Design review of the part built by this model. Coordinates are the model's own, in mm. A direction names the side the tool comes from. Round coordinates to 2 decimals unless told otherwise and drop trailing zeros. Write each loop counter-clockwise with the first axis right and the second up, starting at its lowest first coordinate (ties: lowest second). Pieces come first, ordered by that corner, then holes. Notation, with made-up numbers: (6, -32) -> (21, -32) arc R17 ccw to (21, -18) -> close; hole circle Ø9 at (46.5, 22). An arc over 180 degrees is marked (long way). Write item = value, one per line. Start each with the question number.
Item 1: For pin 1 Ø1.5 at (x, z) = (23, 2) entering from +Y; pin 2 Ø1.9 at (x, z) = (122, 4.5) entering from +Y; pin 3 Ø5.5 at (x, y) = (147.955, 6.35) entering from -Z, all flat-tipped, find the tip position at first contact; note any pin that passes through.
Item 2: Add section C-C, the plane z = 4.5. State the section outline as (x, y) points (3 decimals).
Item 3: To check wall thickness, follow L1, parallel to Y at x = 139.7, z = 4.5; L2, parallel to Y at x = -20, z = 1.5; L3, parallel to X at y = 12, z = 1.5. State the ranges of each line that lie inside material, in increasing order.
Item 4: Machinability: for faces 1 (the flat face through (152.4, -44, 3)), 2 (the flat face through (110, 12.7, 3)), 3 (the flat face through (-111, 12.7, 3)), which of the approach directions +Z, -Z, +X, -X, +Y, -Y give a long, thin tool a straight path to every point of the face, cutting with its end or side? Answer none if there is none.
Item 5: Mouldability with a two-part tool opening along Y and no side actions: class faces 4 (the flat face through (-152.4, -45, 3)), 5 (the cylindrical face through (21.199, 6.676, 3.131)), 6 (the cylindrical face through (41.16, 16.5, 3.13)) as released by +Y, released by -Y, zero draft, split by the parting line, or undercut.
Item 6: Add section A-A, the plane x = 0. State the section outline as (y, z) points (3 decimals).
Item 7: Add section D-D, the plane x = -118. State the section outline as (y, z) points.
Item 8: Add section B-B, the plane y = 0. State the section outline as (x, z) points (3 decimals).
from build123d import *

# Parameters (mm, degrees)
SKETCH1_R           = 22.225
BOSS_EXTRUDE1_DEPTH = 6.35
SKETCH2_R           = 2.159
CUT_EXTRUDE1_DEPTH  = 7.35


with BuildPart() as part:
    # Sketch1 → Boss-Extrude1 (new body)
    with BuildSketch(Plane.XY):
        with BuildLine():
            Line((-152.4, 12.7), (-68.685751798, 12.7))
            ThreePointArc((-68.685751798, 12.7), (-41.532009619, 16.395790255), (-16.353750428, 27.214285714))
            ThreePointArc((-16.353750428, 27.214285714), (0, 31.75), (16.353750428, 27.214285714))
            ThreePointArc((16.353750428, 27.214285714), (41.532009619, 16.395790255), (68.685751798, 12.7))
            Line((68.685751798, 12.7), (152.4, 12.7))
            Line((152.4, 12.7), (152.4, -101.6))
            Line((152.4, -101.6), (-152.4, -101.6))
            Line((-152.4, -101.6), (-152.4, 12.7))
        make_face()
        Circle(SKETCH1_R, mode=Mode.SUBTRACT)
    extrude(amount=BOSS_EXTRUDE1_DEPTH)

    # Sketch2 → Cut-Extrude1 (cut, through all)
    with BuildSketch(Plane.XY.offset(6.35)):
        with Locations((-139.7, -97.155)):
            Circle(SKETCH2_R)
        with Locations((-147.955, 6.35)):
            Circle(SKETCH2_R)
        with Locations((147.955, 6.35)):
            Circle(SKETCH2_R)
        with Locations((139.7, -97.155)):
            Circle(SKETCH2_R)
    extrude(amount=-CUT_EXTRUDE1_DEPTH, mode=Mode.SUBTRACT)


solid = part.part
Result set:
q1.pin_1 = 23.93
q1.pin_2 = 12.7
q1.pin_3 = 0
q2.outline = (-152.4, -101.6) -> (152.4, -101.6) -> (152.4, 12.7) -> (68.686, 12.7) arc R101.6 cw to (16.354, 27.214) arc R31.75 ccw to (-16.354, 27.214) arc R101.6 cw to (-68.686, 12.7) -> (-152.4, 12.7) -> close; hole circle Ø4.318 at (-147.955, 6.35); hole circle Ø4.318 at (-139.7, -97.155); hole circle Ø44.45 at (0, 0); hole circle Ø4.318 at (139.7, -97.155); hole circle Ø4.318 at (147.955, 6.35)
q3.L1 = -101.6 to -99.31, -95 to 12.7
q3.L2 = -101.6 to -9.69, 9.69 to 25.12
q3.L3 = -152.4 to -18.71, 18.71 to 152.4
q4.face_1 = +Z, -Z, +X, +Y, -Y
q4.face_2 = +Z, -Z, +X, +Y
q4.face_3 = +Z, -Z, -X, +Y
q5.face_4 = zero draft
q5.face_5 = undercut
q5.face_6 = released by +Y
q6.outline = (-101.6, 0) -> (-22.225, 0) -> (-22.225, 6.35) -> (-101.6, 6.35) -> close; (22.225, 0) -> (31.75, 0) -> (31.75, 6.35) -> (22.225, 6.35) -> close
q7.outline = (-101.6, 0) -> (12.7, 0) -> (12.7, 6.35) -> (-101.6, 6.35) -> close
q8.outline = (-152.4, 0) -> (-22.225, 0) -> (-22.225, 6.35) -> (-152.4, 6.35) -> close; (22.225, 0) -> (152.4, 0) -> (152.4, 6.35) -> (22.225, 6.35) -> close
